Could you check a few things on this drawing? It's one solid part, dimensions in mm from its lowest x, y, z. A direction names the side the tool comes from. Give positions to 0.01 mm unless a question says otherwise; leave off trailing zeros. Write each loop counter-clockwise with the first axis right and the second up, starting at its lowest first coordinate (ties: lowest second). Pieces come first, ordered by that corner, then holes. Notation, with made-up numbers: (89.5, 29) - (101.5, 29) arc R24 cw to (101.5, 54) - close; hole circle Ø4 at (-10, 61.25). An arc over 180 degrees is marked (long way). One line per item, written item: value. Start each with the question number.
1) We'd pull the mould along X, two halves only. Please class the marked faces 1, 2 and 3: +X half, -X half, draft (parallel to the pull), parting line (faces both ways), or undercut.
2) I'm going to push flat-ended pins straight in: P1, Ø2, axis at x = 7.5, y = 6, coming from the -Z side; P2, Ø1, axis at y = 3.5, z = 9, coming from the +X side; P3, Ø3, axis at x = 6.25, y = 6.25, coming from the +Z side. Where does each tip first touch, or does it pass through?
3) On a 3-axis mill with a long thin cutter (end or side, diameter ignored), from which of +Z, -Z, +X, -X, +Y, -Y can I reach the whole of each face in a straight line? I mean the marked faces 4 and 5. Say none if no direction works.
4) Imagine slicing it at A-A on x = 6.25. Write out the boundary of the cut face in (y, z) (3 decimals).
5) Imagine slicing it at B-B on z = 12. Write out the boundary of the cut face in (x, y), plus the area to 3 significant figures.
6) Imagine slicing it at D-D on z = 6.5. Write out the boundary of the cut face in (x, y), plus the area to 3 significant figures.
7) Please list where these lines run through material, in increasing order: L1, parallel to Y at x = 6.25, z = 2.7 (3 decimals); L2, parallel to Z at x = 4.5, y = 4; L3, parallel to Y at x = 8.75, z = 3. Write a range as [from, to].
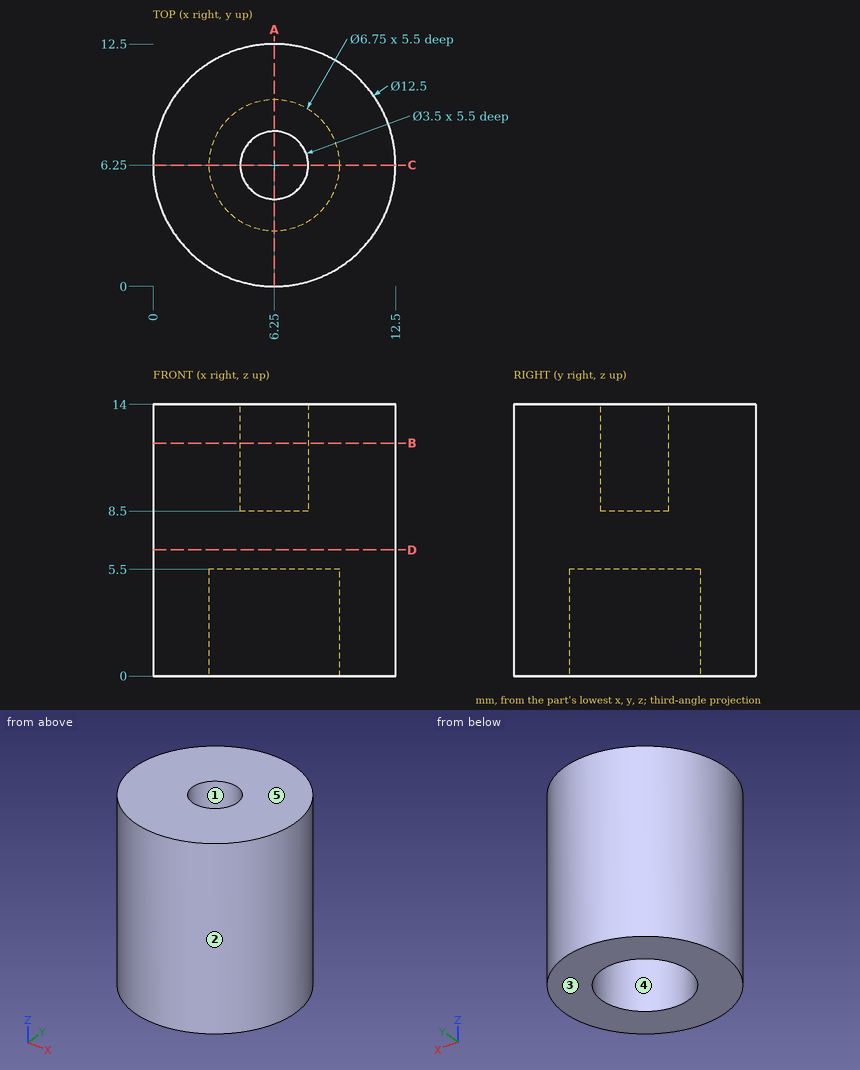
Numbers:
1. face 1: undercut
1. face 2: parting line
1. face 3: draft
2. P1: z = 5.5
2. P2: x = 12.08
2. P3: z = 8.5
3. face 4: -Z
3. face 5: +Z, +X, -X, +Y, -Y
4. outline: (0, 0) - (2.875, 0) - (2.875, 5.5) - (9.625, 5.5) - (9.625, 0) - (12.5, 0) - (12.5, 14) - (8, 14) - (8, 8.5) - (4.5, 8.5) - (4.5, 14) - (0, 14) - close
5. outline: circle Ø12.5 at (6.25, 6.25); hole circle Ø3.5 at (6.25, 6.25)
5. area: 113 mm^2
6. outline: circle Ø12.5 at (6.25, 6.25)
6. area: 123 mm^2
7. L1: [0, 2.875], [9.625, 12.5]
7. L2: [5.5, 14]
7. L3: [0.52, 3.98], [8.52, 11.98]
